Part print with two shaded views. Sizes in mm from the minimum x, y, z corner. A direction names the side the tool comes from. Coordinates: 2 decimals unless noted, no trailing zeros. Write each loop counter-clockwise with the first axis right and the second up, starting at its lowest first coordinate (ties: lowest second). Pieces come first, ordered by that corner, then holes. Notation, with made-up numbers: (71.5, 74.25) - (129.5, 74.25) arc R18 ccw to (129.5, 94.25) - close; hole circle Ø6 at (-35, 86.5). An arc over 180 degrees is marked (long way). One line per question, with ' | ' between items. Start each with the question number.
1. Flat gauge pins, fed straight in: P1, Ø4, axis at x = 59.5, y = 2.5, coming from the -Z side; P2, Ø2.5, axis at x = 57.5, y = 2, coming from the +Z side. Where does each tip first touch, or does it go through?
2. Two-plate mould, pull along Z, no slides. Class the marked faces 4, 5 and 6: +Z half, -Z half, draft (parallel to the pull), parting line (faces both ways), or undercut.
3. Probe line 1 (Y direction, x = 60, z = 34); line 2 (X direction, y = 7.75, z = 42.5). List the from-to ranges inside material, lowest first.
4. Band-saw the part on D-D, the plane z = 4. Write the cut outline in (x, y), then the cut area to 3 significant figures.
5. Band-saw the part on A-A, the plane x = 40. Write the cut outline in (y, z).
6. Which spindle directions (+Z, -Z, +X, -X, +Y, -Y) get a long thin tool onto all of the face, cutting with end or side? Do the marked faces 1, 2 and 3. Say none if no direction does.
7. Band-saw the part on B-B, the plane y = 4. Give the number of separate pieces and of enclosed holes in the cut face, then the cut area to 3 significant figures.
8. Band-saw the part on C-C, the plane x = 60. Write the cut outline in (y, z).
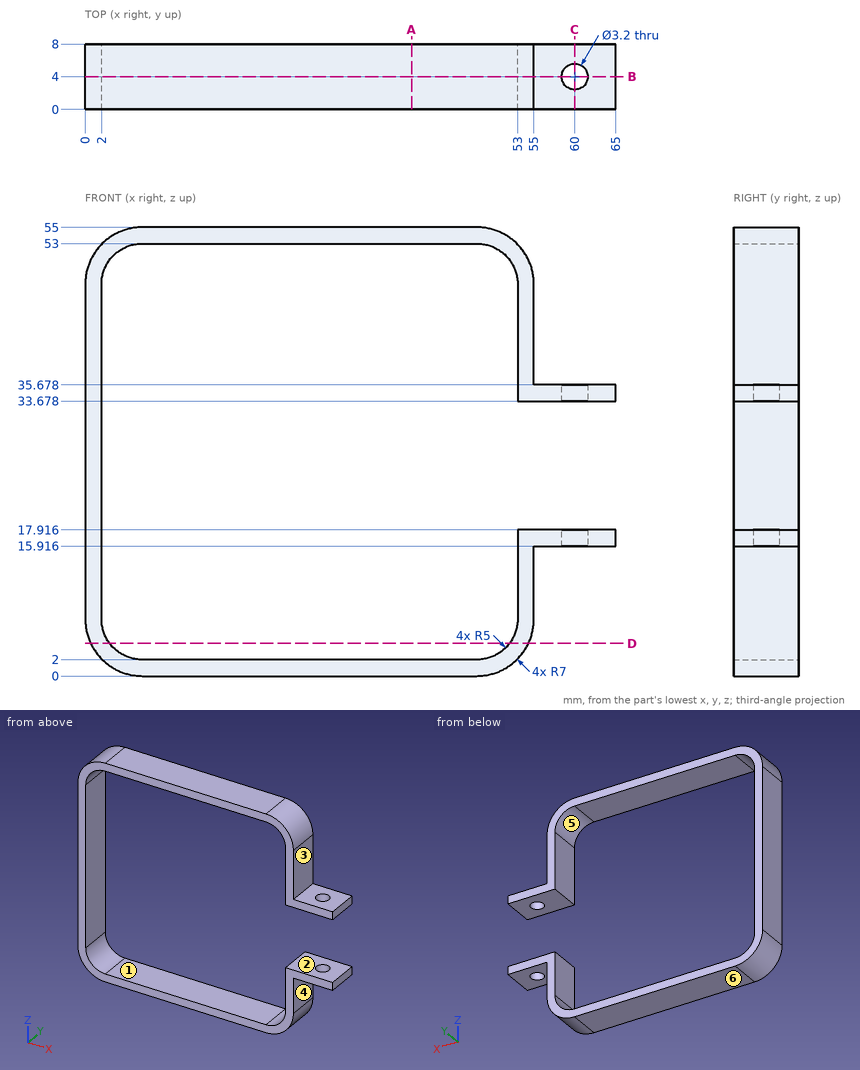
Filled in:
1) P1: stops at z = 15.92 | P2: stops at z = 35.68
2) face 4: draft | face 5: undercut | face 6: -Z half
3) line 1: y = 0 to 2.4, 5.6 to 8 | line 2: x = 0 to 2, 53 to 55
4) outline: (0.68, 0) - (3, 0) - (3, 8) - (0.68, 8) - close; (52, 0) - (54.32, 0) - (54.32, 8) - (52, 8) - close | area: 37.2 mm²
5) outline: (0, 0) - (8, 0) - (8, 2) - (0, 2) - close; (0, 53) - (8, 53) - (8, 55) - (0, 55) - close
6) face 1: +Y, -Y | face 2: +X, +Y, -Y | face 3: +Z, +X, +Y, -Y
7) separate pieces: 3 | enclosed holes: 0 | area: 399 mm²
8) outline: (0, 15.92) - (2.4, 15.92) - (2.4, 17.92) - (0, 17.92) - close; (0, 33.68) - (2.4, 33.68) - (2.4, 35.68) - (0, 35.68) - close; (5.6, 15.92) - (8, 15.92) - (8, 17.92) - (5.6, 17.92) - close; (5.6, 33.68) - (8, 33.68) - (8, 35.68) - (5.6, 35.68) - close
